For this review, take the finished solid that the model builds, in its own axes (mm). Round coordinates to 2 decimals unless told otherwise and drop trailing zeros. Write each loop counter-clockwise with the first axis right and the second up, starting at its lowest first coordinate (ties: lowest second). Pieces come first, ordered by that corner, then holes.
from build123d import *

# Parameters (mm, degrees)
SKETCH1_W                = 234.4674
SKETCH1_H                = 398.9197
BOSS_EXTRUDE1_DEPTH      = 1.5875
BOSS_EXTRUDE2_DEPTH      = 0.0254
BOSS_EXTRUDE2_DEPTH_BACK = 1.6254
SKETCH5_R                = 1.6
CUT_EXTRUDE1_DEPTH       = 2.6254
SKETCH6_W                = 18.565945636
SKETCH6_H                = 24.802104659
BOSS_EXTRUDE3_DEPTH      = 0.1
SKETCH8_R                = 1.6
CUT_EXTRUDE2_DEPTH       = 2.6254
SKETCH7_R                = 1.6
CUT_EXTRUDE3_DEPTH       = 10


with BuildPart() as part:
    # Sketch1 → Boss-Extrude1 (new body)
    with BuildSketch(Plane.XY):
        with Locations((0, -141.80185)):
            Rectangle(SKETCH1_W, SKETCH1_H)
    extrude(amount=BOSS_EXTRUDE1_DEPTH)

    # Sketch4 → Boss-Extrude2 (add, two sides)
    with BuildSketch(Plane.XY.offset(1.5875)) as boss_extrude2_sk:
        Polygon((-117.2337, 5.08), (117.2337, 5.08), (117.2337, -5.08), (22.987, -5.08), (22.987, -341.2617), (12.827, -341.2617), (12.827, -5.08), (-117.2337, -5.08), align=None)
    extrude(amount=BOSS_EXTRUDE2_DEPTH)
    extrude(boss_extrude2_sk.sketch, amount=-BOSS_EXTRUDE2_DEPTH_BACK)

    # Sketch5 → Cut-Extrude1 (cut, through all)
    with BuildSketch(Plane.XY.offset(1.5875)):
        with Locations((112.2337, 43.514)):
            Circle(SKETCH5_R)
        with Locations((112.2337, -327.1177)):
            Circle(SKETCH5_R)
    cut_extrude1 = extrude(amount=-CUT_EXTRUDE1_DEPTH, mode=Mode.SUBTRACT)

    # Mirror3: Cut-Extrude1 across plane
    add(cut_extrude1.mirror(Plane(origin=(0, 0, 0), x_dir=(0, 0, 1), z_dir=(1, 0, 0))), mode=Mode.SUBTRACT)

    # Sketch6 → Boss-Extrude3 (add)
    with BuildSketch(Plane.XY.offset(1.5875)):
        with Locations((-96.012, -328.860647671)):
            Rectangle(SKETCH6_W, SKETCH6_H)
    extrude(amount=BOSS_EXTRUDE3_DEPTH)

    # Sketch8 → Cut-Extrude2 (cut, through all)
    with BuildSketch(Plane.XY.offset(1.5875)):
        with Locations((-114.2337, 22.85873)):
            Circle(SKETCH8_R)
        with Locations((-114.2337, -13.33627)):
            Circle(SKETCH8_R)
    extrude(amount=-CUT_EXTRUDE2_DEPTH, mode=Mode.SUBTRACT)

    # Sketch7 → Cut-Extrude3 (cut)
    with BuildSketch(Plane.XY.offset(1.5875)):
        with Locations((-112.2337, -31.486)):
            Circle(SKETCH7_R)
    extrude(amount=-CUT_EXTRUDE3_DEPTH, mode=Mode.SUBTRACT)


solid = part.part
(1) We need section D-D, the plane y = 9. Give the boundary of the cut face in (x, z).
Geometry check:
outline: (-117.23, 0) - (117.23, 0) - (117.23, 1.59) - (-117.23, 1.59) - close
(2) For line 1 along Z through (x, y) = (-66.5, 3.5), list the stretches that pass through material, from the lowest coordinate up.
Geometry check:
line 1: z = -0.04 to 1.61
(3) For pin 1 Ø1.5 at (x, y) = (-48, -69.5) entering from -Z; pin 2 Ø1.9 at (x, y) = (-112.23, -327.12) entering from +Z; pin 3 Ø10 at (x, y) = (-8.5, -7.5) entering from +Z, all flat-tipped, find the tip position at first contact; note any pin that passes through.
Geometry check:
pin 1: stops at z = 0
pin 2: passes through
pin 3: stops at z = 1.61
